Build history of the part. All positions in model axes, mm. A direction names the side the tool comes from. Give positions to 0.01 mm unless a question says otherwise; leave off trailing zeros. Use a Markdown table: item, result.
from build123d import *

# Parameters (mm, degrees)
SKETCH_R        = 70
SKETCH_R_2      = 57.25
PAD_DEPTH       = 15
SKETCH001_R     = 4
SKETCH002_W     = 40
SKETCH002_H     = 40
PAD001_DEPTH    = 5
SKETCH003_R     = 2.5
POCKET_DEPTH    = 5
FILLET_R        = 18
FILLET001_R     = 11
SKETCH004_R     = 58
POCKET001_DEPTH = 15.001


with BuildPart() as part:
    # Sketch → Pad (new body)
    with BuildSketch(Plane.XY):
        Circle(SKETCH_R)
        Circle(SKETCH_R_2, mode=Mode.SUBTRACT)
    extrude(amount=PAD_DEPTH)

    # Sketch001 → Groove (revolve, cut)
    with BuildSketch(Plane.XZ):
        with Locations((63.625, 16)):
            Circle(SKETCH001_R)
    revolve(axis=Axis((0, 0, 0), (0, 0, 1)), mode=Mode.SUBTRACT)

    # Sketch002 (on Face2 of Groove) → Pad001 (join)
    with BuildSketch(Plane(origin=(0, 0, 0), x_dir=(1, 0, 0), z_dir=(0, 0, -1))):
        with Locations((82, 0)):
            Rectangle(SKETCH002_W, SKETCH002_H)
        with Locations((-82, 0)):
            Rectangle(SKETCH002_W, SKETCH002_H)
        with Locations((0, 82)):
            Rectangle(SKETCH002_W, SKETCH002_H)
        with Locations((0, -82)):
            Rectangle(SKETCH002_W, SKETCH002_H)
    extrude(amount=-PAD001_DEPTH)

    # Sketch003 (on Face13 of Pad001) → Pocket (cut)
    with BuildSketch(Plane.XY.offset(5)):
        with Locations((-86.25, 0)):
            Circle(SKETCH003_R)
        with Locations((0, -86.25)):
            Circle(SKETCH003_R)
        with Locations((86.25, 0)):
            Circle(SKETCH003_R)
        with Locations((0, 86.25)):
            Circle(SKETCH003_R)
    extrude(amount=-POCKET_DEPTH, mode=Mode.SUBTRACT)

    # Fillet
    fillet_edges = [part.edges().sort_by_distance(p)[0] for p in [
        (-20, 102, 2.5),
        (20, 102, 2.5),
        (102, 20, 2.5),
        (102, -20, 2.5),
        (20, -102, 2.5),
        (-20, -102, 2.5),
        (-102, -20, 2.5),
        (-102, 20, 2.5),
    ]]
    fillet(fillet_edges, radius=FILLET_R)

    # Fillet001
    fillet001_edges = [part.edges().sort_by_distance(p)[0] for p in [
        (67.082039, 20, 2.5),
        (20, 67.082039, 2.5),
        (-20, 67.082039, 2.5),
        (-67.082039, 20, 2.5),
        (-67.082039, -20, 2.5),
        (-20, -67.082039, 2.5),
        (20, -67.082039, 2.5),
        (67.082039, -20, 2.5),
    ]]
    fillet(fillet001_edges, radius=FILLET001_R)

    # Sketch004 (on Face41 of Fillet001) → Pocket001 (cut, through all)
    with BuildSketch(Plane.XY.offset(15)):
        Circle(SKETCH004_R)
    extrude(amount=-POCKET001_DEPTH, mode=Mode.SUBTRACT)


solid = part.part
1) Wall check: line 1 (Z direction, x = -83, y = -4); line 2 (X direction, y = 18.5, z = 14); line 3 (Y direction, x = -86.25, z = 1.4). Give the ranges that are in metal, low to high. Write a range as from..to.
Computed:
| item | result |
|---|---|
| line 1 | z = 0..5 |
| line 2 | x = -67.51..-64.49, -57.25..-54.97, 54.97..57.25, 64.49..67.51 |
| line 3 | y = -19.86..-2.5, 2.5..19.86 |
2) Pin check, flat tips, straight feed: P1, Ø11, axis at x = 77.5, y = 11, coming from the +Z side; P2, Ø5.5, axis at x = -78, z = 1.5, coming from the +Y side; P3, Ø4, axis at x = -60, z = 8, coming from the -Y side; P4, Ø6, axis at x = -86.25, y = 0, coming from the -Z side. Stop position of each tip, or through.
Computed:
| item | result |
|---|---|
| P1 | stops at z = 5 |
| P2 | stops at y = 20 |
| P3 | stops at y = -39.19 |
| P4 | stops at z = 0 |
3) Two-plate mould, pull along Y, no slides. Class faces 4 (the cylindrical face through (-14.587, 96.867, 2.535)), 5 (the flat face through (20, 79, 2)), 6 (the cylindrical face through (-68.65, -21.9, 2.46)), 7 (the cylindrical face through (83.752, 0.11, 2.535)): +Y half, -Y half, draft (parallel to the pull), parting line (faces both ways), or undercut.
Computed:
| item | result |
|---|---|
| face 4 | +Y half |
| face 5 | draft |
| face 6 | -Y half |
| face 7 | undercut |
4) Tool access for faces 1 (the flat face through (79, -20, 2)), 2 (the flat face through (-20, 79, 2)), 3 (the cylindrical face through (-88.748, 0.11, 2.535)): list every direction of +Z, -Z, +X, -X, +Y, -Y with a clear straight run to the whole face (end or side of a thin tool).
Computed:
| item | result |
|---|---|
| face 1 | +Z, -Z, +X, -Y |
| face 2 | +Z, -Z, -X, +Y |
| face 3 | +Z, -Z |
